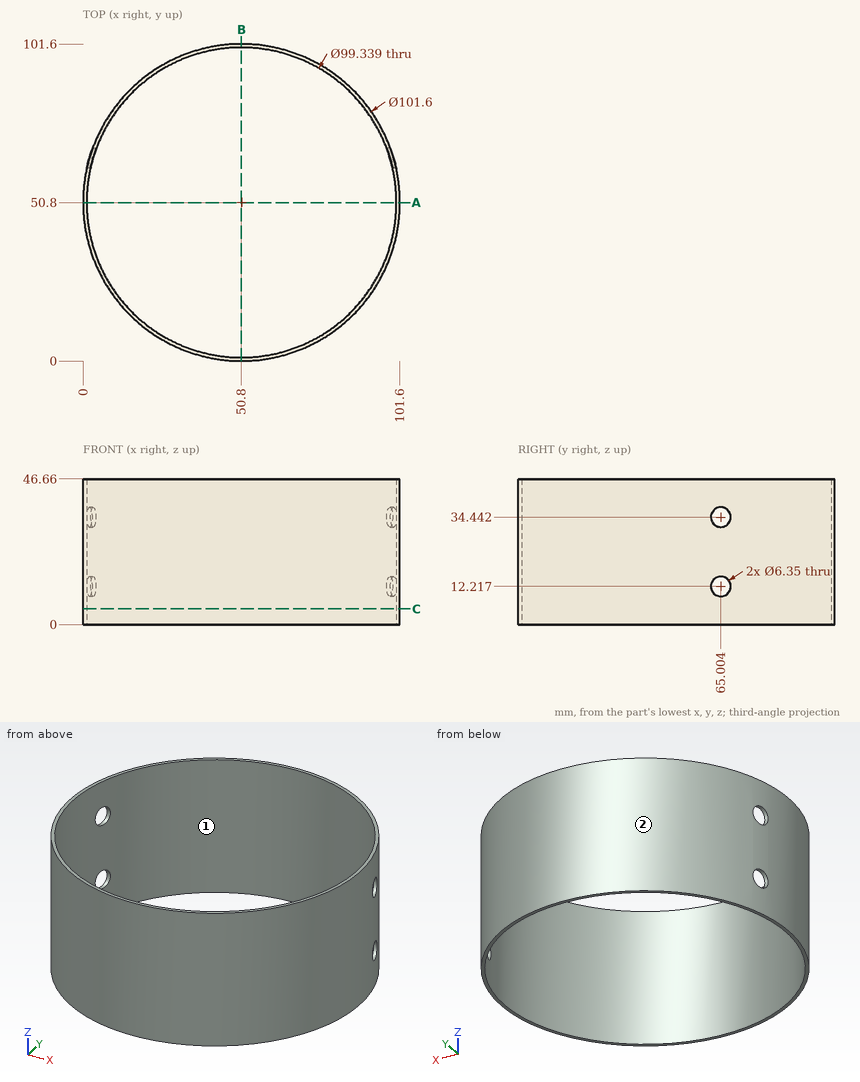
The drawing under review shows one solid part. Ordinate dimensions are in mm from its lowest x, y, z. Round coordinates to 2 decimals unless told otherwise and drop trailing zeros. Write each loop counter-clockwise with the first axis right and the second up, starting at its lowest first coordinate (ties: lowest second). Pieces come first, ordered by that corner, then holes. Notation, with made-up numbers: (-39.75, -22) -> (-3.75, -22) arc R32 cw to (-3.75, 4) -> close; hole circle Ø5 at (40.25, 61). An arc over 180 degrees is marked (long way). One line per question, with ' | ' between items. Start each with the question number.
(1) Add section A-A, the plane y = 50.8. Write out the cut boundary in (x, z).
(2) Insertion check: P1, Ø10, axis at y = 65, z = 34.44, coming from the -X side; P2, Ø8.5, axis at y = 65, z = 12.22, coming from the -X side; P3, Ø1, axis at x = 36, z = 27.5, coming from the -Y side (1 decimal). Each pin has a flat end and moves straight along its axis. Give the tip position at first contact, or say it passes through.
(3) Add section C-C, the plane z = 5. Write out the cut boundary in (x, y).
(4) Mouldability with a two-part tool opening along Y and no side actions: class the marked faces 1 and 2 as released by +Y, released by -Y, zero draft, split by the parting line, or undercut.
(5) For line 1 along X through (y, z) = (51.5, 6) (1 decimal); line 2 along Y through (x, z) = (77, 30); line 3 along Y through (x, z) = (43, 41.5), list the stretches that pass through material, from the lowest coordinate up. Write a range as from..to.
Answer list:
1) outline: (0, 0) -> (1.13, 0) -> (1.13, 46.66) -> (0, 46.66) -> close; (100.47, 0) -> (101.6, 0) -> (101.6, 46.66) -> (100.47, 46.66) -> close
2) P1: x = 0.84 | P2: x = 0.98 | P3: y = 2.1
3) outline: circle Ø101.6 at (50.8, 50.8); hole circle Ø99.34 at (50.8, 50.8)
4) face 1: undercut | face 2: split by the parting line
5) line 1: 0..1.1, 100.5..101.6 | line 2: 7.28..8.6, 93..94.32 | line 3: 0.6..1.75, 99.85..101
